Part model, mm, in its own coordinate system. Round coordinates to 2 decimals unless told otherwise and drop trailing zeros. Loops run counter-clockwise (first coordinate to the right, second up) from the corner with the lowest first, then second, coordinate; pieces in that order, holes last.
from build123d import *

# Parameters (mm, degrees)
SKETCH1_R                = 2.38125
BOSS_EXTRUDE1_DEPTH      = 225.425
BOSS_EXTRUDE1_DEPTH_BACK = 225.425


with BuildPart() as part:
    # Sketch1 → Boss-Extrude1 (new body, two sides)
    with BuildSketch(Plane(origin=(0, 0, 0), x_dir=(0, 0, -1), z_dir=(1, 0, 0))) as boss_extrude1_sk:
        with BuildLine():
            Line((7.039054482, 0.508), (3.959468146, 5.842))
            ThreePointArc((3.959468146, 5.842), (3.587586336, 6.21388181), (3.079586336, 6.35))
            Line((3.079586336, 6.35), (-3.079586336, 6.35))
            ThreePointArc((-3.079586336, 6.35), (-3.587586336, 6.21388181), (-3.959468146, 5.842))
            Line((-3.959468146, 5.842), (-7.039054482, 0.508))
            ThreePointArc((-7.039054482, 0.508), (-7.175172672, 0), (-7.039054482, -0.508))
            Line((-7.039054482, -0.508), (-3.959468146, -5.842))
            ThreePointArc((-3.959468146, -5.842), (-3.587586336, -6.21388181), (-3.079586336, -6.35))
            Line((-3.079586336, -6.35), (3.079586336, -6.35))
            ThreePointArc((3.079586336, -6.35), (3.587586336, -6.21388181), (3.959468146, -5.842))
            Line((3.959468146, -5.842), (7.039054482, -0.508))
            ThreePointArc((7.039054482, -0.508), (7.175172672, 0), (7.039054482, 0.508))
        make_face()
        Circle(SKETCH1_R, mode=Mode.SUBTRACT)
    extrude(amount=BOSS_EXTRUDE1_DEPTH)
    extrude(boss_extrude1_sk.sketch, amount=-BOSS_EXTRUDE1_DEPTH_BACK)


solid = part.part
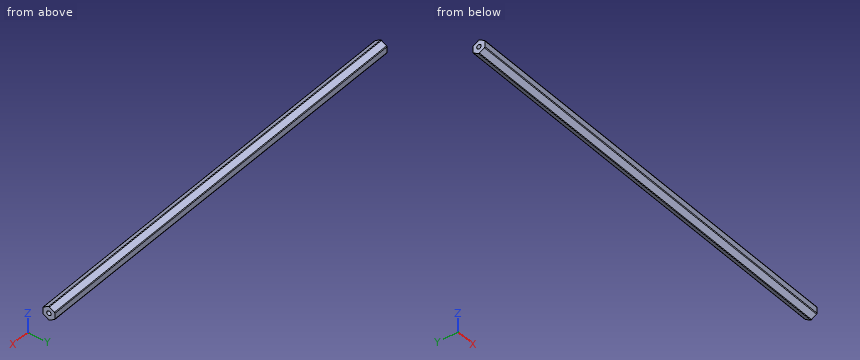
1) Wall check: line 1 along Y through (x, z) = (-11.5, 0); line 2 along Z through (x, y) = (-80.5, -0.25); line 3 along Y through (x, z) = (125, -3.5). Give the ranges that are in metal, low to high.
Values:
line 1: y = -6.35 to -2.38, 2.38 to 6.35
line 2: z = -7.14 to -2.37, 2.37 to 7.14
line 3: y = -6.26 to 6.26
2) Slice it at A-A, the plane x = 147.5. Give the cut face in (y, z).
Values:
outline: (-6.35, -3.08) arc R1.02 ccw to (-5.84, -3.96) - (-0.51, -7.04) arc R1.02 ccw to (0.51, -7.04) - (5.84, -3.96) arc R1.02 ccw to (6.35, -3.08) - (6.35, 3.08) arc R1.02 ccw to (5.84, 3.96) - (0.51, 7.04) arc R1.02 ccw to (-0.51, 7.04) - (-5.84, 3.96) arc R1.02 ccw to (-6.35, 3.08) - close; hole circle Ø4.76 at (0, 0)
3) Slice it at B-B, the plane z = 0. Give the cut face in (x, y) (3 decimals), then the cut area to 3 significant figures.
Values:
outline: (-225.425, -6.35) - (225.425, -6.35) - (225.425, -2.381) - (-225.425, -2.381) - close; (-225.425, 2.381) - (225.425, 2.381) - (225.425, 6.35) - (-225.425, 6.35) - close
area: 3,580 mm2
4) Drop a flat-ended pin along its axis: pin 1 Ø1.5 at (y, z) = (0.5, -1) entering from +X. Give the stop position or say it passes through.
Values:
pin 1: passes through
